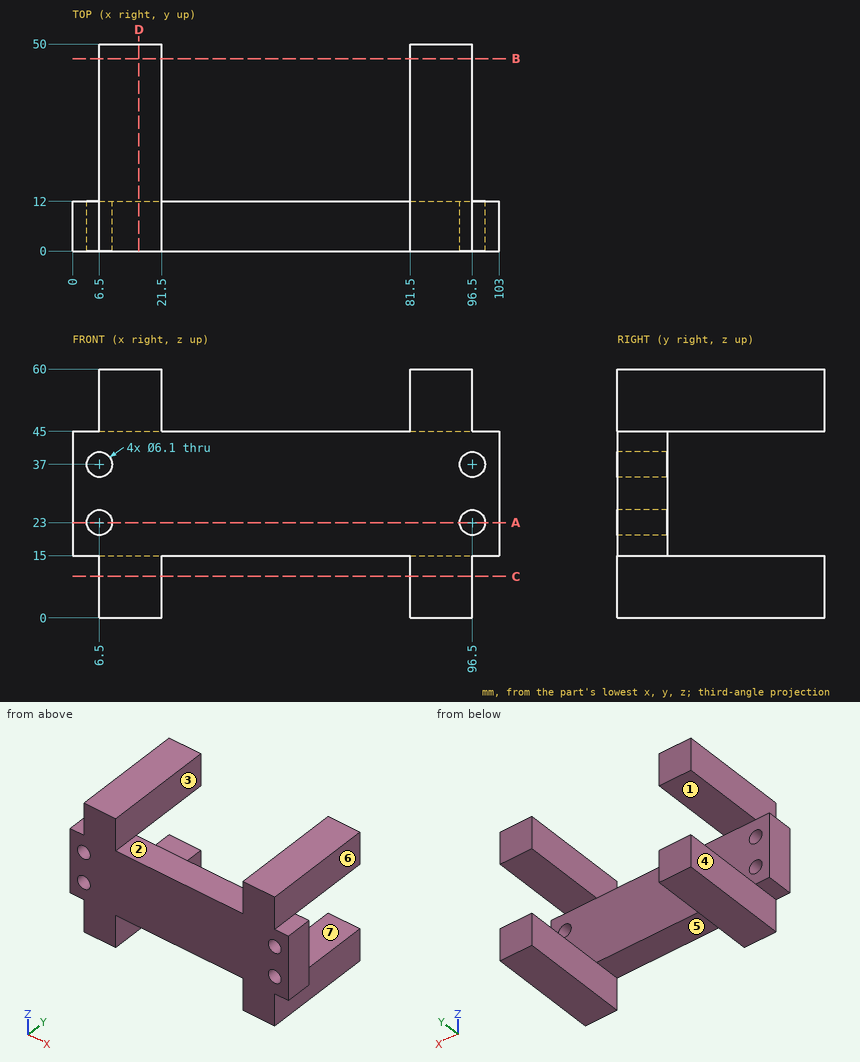
Design review of the part shown in the three views and the two pictorial views. Dimensions are in mm from the part's minimum x, y and z. A direction names the side the tool comes from. Give positions to 0.01 mm unless a question says otherwise; leave off trailing zeros. Order: outer loops, then holes, each group sorted by start corner. A loop starts at its lowest first (then second) coordinate and runs counter-clockwise, first axis right, second up. Notation, with made-up numbers: M 37,-4.5 L 78,-4.5 A32 cw 78,32.5 Z; hole C 53.25,23 d4. An arc over 180 degrees is marked long. Answer in a Markdown table with one row per item. Add a question column.
(1) Consider section A-A on z = 23. State the section outline as (x, y) points.
(2) Wall thickness on probe 1 along X at (y, z) = (5, 37); probe 2 along Z at (x, y) = (86.5, 39); probe 3 along X at (y, z) = (17, 55): over which ranges is each line inside the solid? List them lowest first. Write a range as [from, to].
(3) Mouldability with a two-part tool opening along X and no side actions: class the marked faces 1, 2, 3 and 4 as +X half, -X half, draft (parallel to the pull), parting line (faces both ways), or undercut.
(4) For pin 1 (4.5 mm diameter, centred on y = 20.5, z = 52, fed in from +X); pin 2 (9.5 mm diameter, centred on x = 60, y = 4.5, fed in from +Z); pin 3 (5 mm diameter, centred on x = 4.5, y = 7.5, fed in from +Z); pin 4 (12 mm diameter, centred on x = 65, z = 48.5, fed in from +Y), all flat-tipped, find the tip position at first contact; note any pin that passes through.
(5) For the marked faces 5, 6 and 7, list the 3-axis set-ups (+Z, -Z, +X, -X, +Y, -Y) from which the entire face can be reached by the end or side of a thin tool; tool diameter is ignored.
(6) Consider section B-B on y = 46.5. State the section outline as (x, z) points, and give its area (3 significant figures).
(7) Consider section D-D on x = 16. State the section outline as (y, z) points.
(8) Consider section C-C on z = 10. State the section outline as (x, y) points.
Evaluation:
| question | item | result |
|---|---|---|
| 1 | outline | M 0,0 L 3.45,0 L 3.45,12 L 0,12 Z; M 9.55,0 L 93.45,0 L 93.45,12 L 9.55,12 Z; M 99.55,0 L 103,0 L 103,12 L 99.55,12 Z |
| 2 | probe 1 | x = [0, 3.45], [9.55, 93.45], [99.55, 103] |
| 2 | probe 2 | z = [0, 15], [45, 60] |
| 2 | probe 3 | x = [6.5, 21.5], [81.5, 96.5] |
| 3 | face 1 | draft |
| 3 | face 2 | undercut |
| 3 | face 3 | undercut |
| 3 | face 4 | -X half |
| 4 | pin 1 | stops at x = 96.5 |
| 4 | pin 2 | stops at z = 45 |
| 4 | pin 3 | stops at z = 60 |
| 4 | pin 4 | stops at y = 12 |
| 5 | face 5 | -Z, +Y, -Y |
| 5 | face 6 | +Z, +X, +Y, -Y |
| 5 | face 7 | +X, -X, +Y |
| 6 | outline | M 6.5,0 L 21.5,0 L 21.5,15 L 6.5,15 Z; M 6.5,45 L 21.5,45 L 21.5,60 L 6.5,60 Z; M 81.5,0 L 96.5,0 L 96.5,15 L 81.5,15 Z; M 81.5,45 L 96.5,45 L 96.5,60 L 81.5,60 Z |
| 6 | area | 900 mm^2 |
| 7 | outline | M 0,0 L 50,0 L 50,15 L 12,15 L 12,45 L 50,45 L 50,60 L 0,60 Z |
| 8 | outline | M 6.5,0 L 21.5,0 L 21.5,50 L 6.5,50 Z; M 81.5,0 L 96.5,0 L 96.5,50 L 81.5,50 Z |
